Read the model definition and answer for the solid it produces. Units are mm, in the model's axes. Face numbers are marked on the shaded views. A direction names the side the tool comes from. Coordinates: 2 decimals unless noted, no trailing zeros. One line per item, written item: value. Start each with the question number.
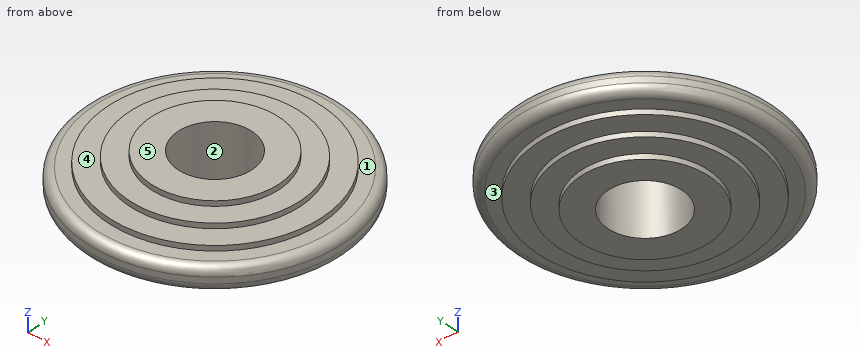
```python
from build123d import *

# Parameters (mm, degrees)
F0_R      = 38.1
F1_DEPTH  = 6.9342
F2_R      = 2.54
F3_R      = 31.75
F4_DEPTH  = 1.524
F6_R      = 19.05
F7_DEPTH  = 1.524
F5_R      = 25.4
F8_DEPTH  = 1.524
F9_R      = 19.05
F10_DEPTH = 1.524
F11_R     = 31.75
F12_DEPTH = 1.524
F13_R     = 25.4
F14_DEPTH = 1.524
F15_R     = 19.05
F16_DEPTH = 1.524
F17_R     = 10.9728
F18_DEPTH = 25.4


with BuildPart() as f1:
    # F0 (on Top) → F1 (new body)
    with BuildSketch(Plane.XY):
        Circle(F0_R)
    extrude(amount=F1_DEPTH)

    # F2
    f2_edges = [f1.edges().sort_by_distance(p)[0] for p in [
        (-38.1, 0, 6.9342),
        (-38.1, 0, 0),
    ]]
    fillet(f2_edges, radius=F2_R)

    # F3 (on face) → F4 (join)
    with BuildSketch(Plane(origin=(0, 0, 0), x_dir=(1, 0, 0), z_dir=(0, 0, -1))):
        Circle(F3_R)
    extrude(amount=F4_DEPTH)

    # F5 (on face) → F8 (join)
    with BuildSketch(Plane(origin=(0, 0, -1.524), x_dir=(1, 0, 0), z_dir=(0, 0, -1))):
        Circle(F5_R)
    extrude(amount=F8_DEPTH)



with BuildPart() as f7:
    # F6 (on face) → F7 (new body)
    with BuildSketch(Plane.XY.offset(8.4582)):
        Circle(F6_R)
    extrude(amount=F7_DEPTH)

    # F9 (on face) → F10 (join)
    with BuildSketch(Plane.XY.offset(9.9822)):
        Circle(F9_R)
    extrude(amount=F10_DEPTH)


with BuildPart() as f1_1:
    add(f1.part)

    add(f7.part)  # F12 merges F7
    # F11 (on face) → F12 (join)
    with BuildSketch(Plane.XY.offset(6.9342)):
        Circle(F11_R)
    extrude(amount=F12_DEPTH)

    # F13 (on face) → F14 (join)
    with BuildSketch(Plane.XY.offset(8.4582)):
        Circle(F13_R)
    extrude(amount=F14_DEPTH)

    # F15 (on face) → F16 (join)
    with BuildSketch(Plane(origin=(0, 0, -3.048), x_dir=(1, 0, 0), z_dir=(0, 0, -1))):
        Circle(F15_R)
    extrude(amount=F16_DEPTH)

    # F17 (on face) → F18 (cut)
    with BuildSketch(Plane(origin=(0, 0, -4.572), x_dir=(1, 0, 0), z_dir=(0, 0, -1))):
        Circle(F17_R)
    extrude(amount=-F18_DEPTH, mode=Mode.SUBTRACT)


solid = f1_1.part
```
1) Flat-ended cylindrical pins translate along their axes: pin 1 (1 mm diameter, centred on x = 8, z = 2, fed in from -Y); pin 2 (5 mm diameter, centred on y = 28, z = 2, fed in from +X); pin 3 (1 mm diameter, centred on x = 11.5, z = 2.5, fed in from +Y). Find the tip coordinate at first contact, or state that the pin passes through.
2) Consider line 1 along Y through (x, z) = (0, 8); line 2 along Y through (x, z) = (-33, 2.5); line 3 along Z through (x, y) = (-1, 35). Determine where each line is inside the solid, lowest interval first.
3) For a pull along X with two mould halves and no side action, classify the marked faces 1 and 2 as released by +X, released by -X, zero draft, split by the parting line, or undercut.
4) A tool of negligible diameter and unlimited length cuts with its end or side. For the marked faces 3, 4 and 5, from which of +Z, -Z, +X, -X, +Y, -Y can it reach the whole face along a straight path? Write none if from no direction.
Results found:
1. pin 1: stops at y = -37.32
1. pin 2: stops at x = 28.28
1. pin 3: stops at y = 36.48
2. line 1: y = -31.75 to -10.97, 10.97 to 31.75
2. line 2: y = -19.04 to 19.04
2. line 3: z = 0 to 6.93
3. face 1: zero draft
3. face 2: undercut
4. face 3: -Z
4. face 4: +Z
4. face 5: +Z, +X, -X, +Y, -Y
